Geometry: final body of the model. Coordinates: model frame, mm. A direction names the side the tool comes from. Give positions to 0.01 mm unless a question says otherwise; leave off trailing zeros. Loops run counter-clockwise (first coordinate to the right, second up) from the corner with the lowest first, then second, coordinate; pieces in that order, holes last. Notation, with made-up numbers: (76, 23.5) -> (128, 23.5) arc R30 cw to (128, 47.5) -> close; hole circle Ø2 at (44.25, 12). An arc over 180 degrees is marked (long way). Answer in a Markdown table with one row per item. Add a question column.
1) Section query A-A (x = 0). Return the cut outline in (y, z) (3 decimals), plus the area to 3 significant figures.
2) Section query C-C (z = -137). Return the cut outline in (x, y).
3) Section query D-D (z = -68). Return the cut outline in (x, y) (3 decimals).
4) First-contact query: P1, Ø6, axis at y = 5, z = -80, coming from the -X side; P2, Ø6, axis at x = 0, y = 6, coming from the +Z side; P3, Ø5, axis at y = -5, z = -18.5, coming from the -X side. Flat tips, straight axial feed; report the tip coordinate or a pass-through.
5) Access query for faces 1 (the flat face through (-1, 3, -144.35)), 2 (the flat face through (2, -3, -27.8)), 3 (the cylindrical face through (7.607, -2.395, -80.352)). Directions: +Z, -Z, +X, -X, +Y, -Y. A direction counts if a zero-diameter tool reaches every point of the face in a straight line with its end or side. Return the directions, or none.
6) Line query: line 1 (Z direction, x = -4.5, y = 1); line 2 (Z direction, x = 2.5, y = -2.5); line 3 (Y direction, x = -1, z = -123). Output: solid intervals per line, ascending. Write a range as from..to.
```python
from build123d import *


with BuildPart() as part:
    # Esquisse1 → Base-Révolution (revolve)
    with BuildSketch(Plane(origin=(0, 0, 0), x_dir=(0, 0, -1), z_dir=(1, 0, 0)), mode=Mode.PRIVATE) as base_r_volution_sk:
        Polygon((27.8, 3.16), (27.8, 3.95), (36.8, 3.95), (36.8, 6), (51.2, 7.975), (108.7, 7.975), (123.1, 6), (123.1, 3.95), (144.35, 3.95), (144.35, 2.95), (153.85, 2.95), (153.85, 0), (-9.5, 0), (-9.5, 2.95), (0, 2.95), (0, 3.16), align=None)
    revolve(base_r_volution_sk.sketch.rotate(Axis((0, 0, 59.941388175), (0, 0, -1)), 90), axis=Axis((0, 0, 59.941388175), (0, 0, -1)))


solid = part.part
```
Evaluation:
| question | item | result |
|---|---|---|
| 1 | outline | (-7.975, -108.7) -> (-6, -123.1) -> (-3.95, -123.1) -> (-3.95, -144.35) -> (-2.95, -144.35) -> (-2.95, -153.85) -> (2.95, -153.85) -> (2.95, -144.35) -> (3.95, -144.35) -> (3.95, -123.1) -> (6, -123.1) -> (7.975, -108.7) -> (7.975, -51.2) -> (6, -36.8) -> (3.95, -36.8) -> (3.95, -27.8) -> (3.16, -27.8) -> (3.16, 0) -> (2.95, 0) -> (2.95, 9.5) -> (-2.95, 9.5) -> (-2.95, 0) -> (-3.16, 0) -> (-3.16, -27.8) -> (-3.95, -27.8) -> (-3.95, -36.8) -> (-6, -36.8) -> (-7.975, -51.2) -> close |
| 1 | area | 1,850 mm² |
| 2 | outline | circle Ø7.9 at (0, 0) |
| 3 | outline | circle Ø15.95 at (0, 0) |
| 4 | P1 | x = -7.72 |
| 4 | P2 | z = 0 |
| 4 | P3 | x = -1.93 |
| 5 | face 1 | -Z |
| 5 | face 2 | +Z |
| 5 | face 3 | +Z, -Z |
| 6 | line 1 | -123.1..-36.8 |
| 6 | line 2 | -144.35..-27.8 |
| 6 | line 3 | -5.93..5.93 |
